Can you work these out from the model? Positions are in its coordinate system, mm. Give positions to 0.01 mm unless a question says otherwise; leave off trailing zeros. Loops run counter-clockwise (first coordinate to the right, second up) from the corner with the lowest first, then second, coordinate; pieces in that order, holes last. Notation, with made-up numbers: M 18.5,-21 L 72.5,-21 A16 ccw 72.5,-15 Z; hole C 27.25,29 d4. An arc over 180 degrees is marked long. Answer as a JSON object with one key per item and string values.
```python
from build123d import *

# Parameters (mm, degrees)
F0_R     = 1.55
F0_R_2   = 1.6
F0_R_3   = 1.65
F0_R_4   = 1.4
F0_R_5   = 1.25
F0_R_6   = 1.45
F0_R_7   = 1.5
F0_R_8   = 1.3
F0_R_9   = 1.35
F1_DEPTH = 10


with BuildPart() as f1:
    # F0 (on Top) → F1 (new body)
    with BuildSketch(Plane.XY):
        Polygon((-15, 20), (-20, 15), (-20, -20), (20, -20), (20, 20), align=None)
        with Locations((-10, -10)):
            Circle(F0_R, mode=Mode.SUBTRACT)
        with Locations((0, -10)):
            Circle(F0_R_2, mode=Mode.SUBTRACT)
        with Locations((10, -10)):
            Circle(F0_R_3, mode=Mode.SUBTRACT)
        with Locations((-10, 0)):
            Circle(F0_R_4, mode=Mode.SUBTRACT)
        with Locations((-10, 10)):
            Circle(F0_R_5, mode=Mode.SUBTRACT)
        Circle(F0_R_6, mode=Mode.SUBTRACT)
        with Locations((10, 0)):
            Circle(F0_R_7, mode=Mode.SUBTRACT)
        with Locations((0, 10)):
            Circle(F0_R_8, mode=Mode.SUBTRACT)
        with Locations((10, 10)):
            Circle(F0_R_9, mode=Mode.SUBTRACT)
    extrude(amount=F1_DEPTH)


solid = f1.part
```
1) If we mould it in two halves opening along Y, with no side actions, what happens to faces 1 (the flat face through (4, 0, 0)), 2 (the flat face through (3, 20, 5)), 3 (the cylindrical face through (-0.17, 11.29, 4.93))? For each: +Y half, -Y half, draft (parallel to the pull), parting line (faces both ways), or undercut.
Answer list:
{"face 1": "draft", "face 2": "+Y half", "face 3": "undercut"}
2) Suppose I cut it at C-C, the plane z = 7.75. Give the number of separate pieces and of enclosed holes in the cut face, and give its area (3 significant figures).
Answer list:
{"separate pieces": "1", "enclosed holes": "9", "area": "1,530 mm^2"}
3) Please list where these lines run through material, in increasing order: line 1 along Y through (x, z) = (0, 4.25); line 2 along Y through (x, z) = (10, 8); line 3 along X through (y, z) = (-0.5, 3.5). Write a range as from..to.
Answer list:
{"line 1": "-20..-11.6, -8.4..-1.45, 1.45..8.7, 11.3..20", "line 2": "-20..-11.65, -8.35..-1.5, 1.5..8.65, 11.35..20", "line 3": "-20..-11.31, -8.69..-1.36, 1.36..8.59, 11.41..20"}
4) Suppose I cut it at A-A, the plane y = -10. Write out the boundary of the cut face in (x, z).
Answer list:
{"outline": "M -20,0 L -11.55,0 L -11.55,10 L -20,10 Z; M -8.45,0 L -1.6,0 L -1.6,10 L -8.45,10 Z; M 1.6,0 L 8.35,0 L 8.35,10 L 1.6,10 Z; M 11.65,0 L 20,0 L 20,10 L 11.65,10 Z"}
5) Suppose I cut it at B-B, the plane x = 0. Write out the boundary of the cut face in (y, z), and give its area (3 significant figures).
Answer list:
{"outline": "M -20,0 L -11.6,0 L -11.6,10 L -20,10 Z; M -8.4,0 L -1.45,0 L -1.45,10 L -8.4,10 Z; M 1.45,0 L 8.7,0 L 8.7,10 L 1.45,10 Z; M 11.3,0 L 20,0 L 20,10 L 11.3,10 Z", "area": "313 mm^2"}
